```python
from build123d import *

# Parameters (mm, degrees)
SKETCH1_R           = 2.5
SKETCH1_W           = 3.2
SKETCH1_H           = 3.2
BOSS_EXTRUDE1_DEPTH = 10
SKETCH2_3_R         = 2.5
SKETCH2_3_W         = 4.5
SKETCH2_3_H         = 4.5
CUT_EXTRUDE2_DEPTH  = 211.475651798
CUT_EXTRUDE1_DEPTH  = 5


with BuildPart() as part:
    # Sketch1 → Boss-Extrude1 (new body)
    with BuildSketch(Plane.XY):
        with BuildLine():
            Line((50, 10), (-200, 10))
            ThreePointArc((-200, 10), (-210, 0), (-200, -10))
            Line((-200, -10), (50, -10))
            ThreePointArc((50, -10), (60, 0), (50, 10))
        make_face()
        Circle(SKETCH1_R, mode=Mode.SUBTRACT)
        with Locations((-200, 0)):
            Circle(SKETCH1_R, mode=Mode.SUBTRACT)
        with Locations((50, 0)):
            Rectangle(SKETCH1_W, SKETCH1_H, mode=Mode.SUBTRACT)
    extrude(amount=BOSS_EXTRUDE1_DEPTH)

    # Sketch2_3 → Cut-Extrude2 (cut, through all)
    with BuildSketch(Plane.XY.offset(10)):
        with Locations((-12.7, 0)):
            Circle(SKETCH2_3_R)
        with Locations((-12.7, 0)):
            Rectangle(SKETCH2_3_W, SKETCH2_3_H)
        Rectangle(SKETCH2_3_W, SKETCH2_3_H)
        with Locations((12.7, 0)):
            Rectangle(SKETCH2_3_W, SKETCH2_3_H)
        with Locations((-200, 0)):
            Rectangle(SKETCH2_3_W, SKETCH2_3_H)
        with Locations((-200, 0)):
            Circle(SKETCH2_3_R)
        with Locations((-187.3, 0)):
            Rectangle(SKETCH2_3_W, SKETCH2_3_H)
        with Locations((-174.6, 0)):
            Rectangle(SKETCH2_3_W, SKETCH2_3_H)
    extrude(amount=-CUT_EXTRUDE2_DEPTH, mode=Mode.SUBTRACT)

    # Sketch2 → Cut-Extrude1 (cut)
    with BuildSketch(Plane.XY.offset(10)):
        Polygon((15.21, -5), (17.75, -2.46), (17.75, 2.46), (15.21, 5), (-15.21, 5), (-17.75, 2.46), (-17.75, -2.46), (-15.21, -5), align=None)
        Polygon((-172.09, -5), (-169.55, -2.46), (-169.55, 2.46), (-172.09, 5), (-202.51, 5), (-205.05, 2.46), (-205.05, -2.46), (-202.51, -5), align=None)
    extrude(amount=-CUT_EXTRUDE1_DEPTH, mode=Mode.SUBTRACT)


solid = part.part
```
Geometry check sheet. Reference: the model listing, model coordinates, mm. A direction names the side the tool comes from. Round coordinates to 2 decimals unless told otherwise and drop trailing zeros. Return JSON: item names as keys, results as strings. Group by question number.
(1) Set-up check for faces 1 (the face through (-175, -2.25, 3)), 2 (the face through (-169.55, 0, 8)): record each of +Z, -Z, +X, -X, +Y, -Y from which the full face is reachable in a straight line by a thin tool's end or side.
(2) Scan lines: line 1 along X through (y, z) = (0.5, 5.75); line 2 along X through (y, z) = (4.25, 8.25); line 3 along Y through (x, z) = (14.5, 4). Record each from-to range of solid material in increasing order. Write a range as [from, to].
(3) Go/stop test with flat-tipped pins: pin 1 (1.5 mm diameter, centred on y = -4, z = 3.5, fed in from +X); pin 2 (11 mm diameter, centred on x = 7.5, y = 0, fed in from +Z); pin 3 (0.9 mm diameter, centred on y = 2, z = 2.5, fed in from -X); pin 4 (5 mm diameter, centred on x = -189, y = -2, fed in from +Z). Record where each tip stops, or that it passes through.
(4) Mould release check, pull along X, two halves, no side actions. Record for faces 3 (the face through (-210, 0, 5)), 4 (the face through (10.45, 0, 3)), 5 (the face through (-188, -5, 8)): pulls with the +X half, pulls with the -X half, needs draft (parallel to the pull), parting line crosses it, or undercut.
Data:
{
 "1": {"face 1": "+Z, -Z", "face 2": "+Z"},
 "2": {"line 1": "[-209.99, -205.05], [-169.55, -17.75], [17.75, 48.4], [51.6, 59.99]", "line 2": "[-209.05, -203.26], [-171.34, -15.96], [15.96, 59.05]", "line 3": "[-10, -2.25], [2.25, 10]"},
 "3": {"pin 1": "x = 59.46", "pin 2": "z = 10", "pin 3": "x = -209.88", "pin 4": "z = 5"},
 "4": {"face 3": "pulls with the -X half", "face 4": "undercut", "face 5": "undercut"}
}
